CAD build for the part. Positions are in the model's coordinates, mm. A direction names the side the tool comes from. Give positions to 0.01 mm unless a question says otherwise; leave off trailing zeros. Loops run counter-clockwise (first coordinate to the right, second up) from the corner with the lowest first, then second, coordinate; pieces in that order, holes last. Notation, with made-up numbers: M 7.25,84 L 46.25,84 A22 cw 46.25,115 Z; hole C 66,53 d2. An arc over 180 degrees is marked long. One line per question, with ' | ' between items.
```python
from build123d import *

# Parameters (mm, degrees)
SKETCH1_W           = 32
SKETCH1_H           = 17
BOSS_EXTRUDE1_DEPTH = 2.5
SKETCH2_W           = 10
SKETCH2_H           = 5
BOSS_EXTRUDE2_DEPTH = 12
SKETCH3_R           = 1.05
CUT_EXTRUDE1_DEPTH  = 12


with BuildPart() as part:
    # Sketch1 → Boss-Extrude1 (new body)
    with BuildSketch(Plane.XY):
        with Locations((16, -8.5)):
            Rectangle(SKETCH1_W, SKETCH1_H)
    extrude(amount=BOSS_EXTRUDE1_DEPTH)

    # Sketch2 → Boss-Extrude2 (add)
    with BuildSketch(Plane.XY.offset(2.5)):
        with Locations((18, -3)):
            Rectangle(SKETCH2_W, SKETCH2_H)
    extrude(amount=BOSS_EXTRUDE2_DEPTH)

    # Sketch3 → Cut-Extrude1 (cut)
    with BuildSketch(Plane.XY.offset(2.5)):
        with Locations((2.05, -2.5)):
            Circle(SKETCH3_R)
        with Locations((2.05, -14.5)):
            Circle(SKETCH3_R)
    extrude(amount=-CUT_EXTRUDE1_DEPTH, mode=Mode.SUBTRACT)


solid = part.part
```
Item 1: Saw through at D-D on z = 11. Give the cut face in (x, y).
Conclusion:
outline: M 13,-5.5 L 23,-5.5 L 23,-0.5 L 13,-0.5 Z
Item 2: Saw through at A-A on y = -14.5. Give the cut face in (x, z).
Conclusion:
outline: M 0,0 L 1,0 L 1,2.5 L 0,2.5 Z; M 3.1,0 L 32,0 L 32,2.5 L 3.1,2.5 Z
Item 3: 3-axis set-ups, long thin cutter, end or side, ignore diameter. For faces 4 (the flat face through (16, -17, 1)), 5 (the flat face through (23, -3, 8)), 6 (the flat face through (0, -9, 1)), 7 (the flat face through (18, -0.5, 8)), 8 (the flat face through (18, -5.5, 8)): which of +Z, -Z, +X, -X, +Y, -Y reach the whole face in a straight line?
Conclusion:
face 4: +Z, -Z, +X, -X, -Y | face 5: +Z, +X, +Y, -Y | face 6: +Z, -Z, -X, +Y, -Y | face 7: +Z, +X, -X, +Y | face 8: +Z, +X, -X, -Y
Item 4: Drop flat-ended pins along their axis: P1, Ø5, axis at x = 22.5, y = -14.5, coming from the -Z side; P2, Ø1.9, axis at x = 2.05, y = -2.5, coming from the +Z side; P3, Ø1.5, axis at y = -2, z = 10.5, coming from the +X side; P4, Ø8, axis at y = -2, z = 12.5, coming from the -X side. Give the stop position or say it passes through.
Conclusion:
P1: z = 0 | P2: through | P3: x = 23 | P4: x = 13
Item 5: Saw through at C-C on y = -2.5. Give the cut face in (x, z).
Conclusion:
outline: M 0,0 L 1,0 L 1,2.5 L 0,2.5 Z; M 3.1,0 L 32,0 L 32,2.5 L 23,2.5 L 23,14.5 L 13,14.5 L 13,2.5 L 3.1,2.5 Z
Item 6: Saw through at B-B on x = 2.05. Give the cut face in (y, z).
Conclusion:
outline: M -17,0 L -15.55,0 L -15.55,2.5 L -17,2.5 Z; M -13.45,0 L -3.55,0 L -3.55,2.5 L -13.45,2.5 Z; M -1.45,0 L 0,0 L 0,2.5 L -1.45,2.5 Z
Item 7: Drill centre lines: line 1 along Y through (x, z) = (2.05, 2); line 2 along Z through (x, y) = (11, -12); line 3 along X through (y, z) = (-3.25, 5.5). Where is each one in solid material? Low to high. Write a range as [from, to].
Conclusion:
line 1: [-17, -15.55], [-13.45, -3.55], [-1.45, 0] | line 2: [0, 2.5] | line 3: [13, 23]
Item 8: Mould opens along X. For faces 1 (the flat face through (32, -9, 1)), 2 (the cylindrical face through (2.535, -3.432, 1.268)), 3 (the flat face through (13, -3, 8)) say: pulls with the +X half, pulls with the -X half, needs draft (parallel to the pull), parting line crosses it, or undercut.
Conclusion:
face 1: pulls with the +X half | face 2: undercut | face 3: pulls with the -X half
